Source: CAD feature listing. Evaluate the final solid. Frame: model axes, mm. Face numbers are marked on the shaded views. A direction names the side the tool comes from. Coordinates: 2 decimals unless noted, no trailing zeros. Loops run counter-clockwise (first coordinate to the right, second up) from the corner with the lowest first, then second, coordinate; pieces in that order, holes last. Notation, with made-up numbers: (-24.75, 68) - (-20.75, 68) arc R21 ccw to (-20.75, 105) - close; hole circle Ø2 at (85.5, 78). An arc over 180 degrees is marked (long way). Use one line per item in the form item = value. Start each with the question number.
from build123d import *

# Parameters (mm, degrees)
SKETCH1_R           = 1.5875
SKETCH1_R_2         = 1.1303
BOSS_EXTRUDE1_DEPTH = 7.14375
CUT_EXTRUDE2_DEPTH  = 0.79375


with BuildPart() as part:
    # Sketch1 → Boss-Extrude1 (new body)
    with BuildSketch(Plane.XY):
        Polygon((6.35, 1.5875), (9.525, 1.5875), (9.525, 4.224628752), (9.525, 10.562648806), (7.319307862, 9.683908365), (-11.458663934, 2.097115291), (-11.458663934, -3.175), (9.525, -3.175), (9.525, -1.5875), (6.35, -1.5875), align=None)
        Circle(SKETCH1_R, mode=Mode.SUBTRACT)
        with Locations((-8.918663934, -0.301005903)):
            Circle(SKETCH1_R_2, mode=Mode.SUBTRACT)
        with Locations((6.624646204, 5.978899029)):
            Circle(SKETCH1_R_2, mode=Mode.SUBTRACT)
    extrude(amount=BOSS_EXTRUDE1_DEPTH)

    # Sketch3 → Cut-Extrude2 (cut)
    with BuildSketch(Plane.XY.offset(7.14375)):
        Polygon((-8.345148438, 3.659663992), (-5.450582972, -3.504636938), (9.525, -3.219186714), (9.525, 3.382363055), (6.034120938, 1.971956363), (3.430086515, 8.417167728), align=None)
    extrude(amount=-CUT_EXTRUDE2_DEPTH, mode=Mode.SUBTRACT)


solid = part.part
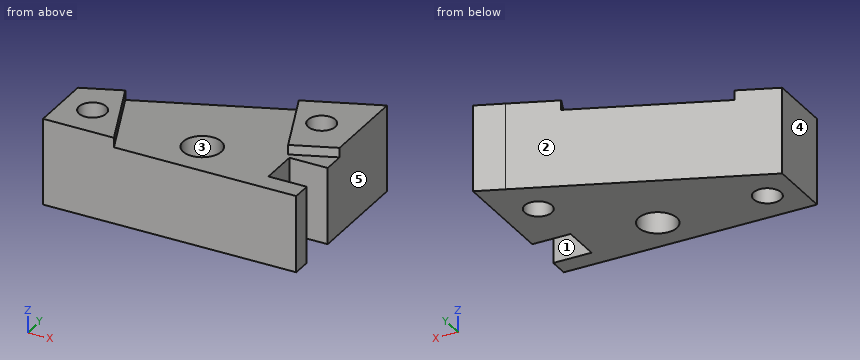
(1) Access query for the marked faces 1 and 2. Directions: +Z, -Z, +X, -X, +Y, -Y. A direction counts if a zero-diameter tool reaches every point of the face in a straight line with its end or side. Return the directions, or none.
(2) Cut plane B-B, the plane y = 0.25. Output: boundary loops of the cut face in (x, z).
(3) Mould query, pull axis X, two halves, no side actions, for the marked faces 3, 4 and 5. Classes: +X half, -X half, draft (parallel to the pull), parting line (faces both ways), or undercut.
(4) Cut plane A-A, the plane z = 6.75. Output: boundary loops of the cut face in (x, y) (3 decimals).
(5) Cut plane D-D, the plane z = 2.25. State how many separate pieces and enclosed holes the cut face has, plus the area to 3 significant figures.
(6) Contact query for flat-ended pins moving along their axis: pin 1 (5.5 mm diameter, centred on x = 4.5, y = 4.5, fed in from +Z); pin 2 (3 mm diameter, centred on x = 2, z = 3, fed in from +Y); pin 3 (1 mm diameter, centred on x = 7.5, z = 4.5, fed in from +Y); pin 4 (2.5 mm diameter, centred on y = 0, z = 3, fed in from +X). Output: stop coordinate, or through.
(7) Material intervals for line 1 (X direction, y = 0, z = 4.25); line 2 (X direction, y = 0.25, z = 1.25); line 3 (Z direction, x = -5.5, y = 0.75), sorted ascending.
Recorded:
q1.face_1 = +Z, -Z, +X
q1.face_2 = +Z, -Z, -X, +Y
q2.outline = (-11.46, 0) - (-9.91, 0) - (-9.91, 7.14) - (-11.46, 7.14) - close; (-7.93, 0) - (-1.57, 0) - (-1.57, 6.35) - (-6.97, 6.35) - (-6.97, 7.14) - (-7.93, 7.14) - close; (1.57, 0) - (6.35, 0) - (6.35, 6.35) - (1.57, 6.35) - close
q3.face_3 = undercut
q3.face_4 = -X half
q3.face_5 = +X half
q4.outline = (-11.459, -3.175) - (-5.584, -3.175) - (-8.239, 3.398) - (-11.459, 2.097) - close; (3.536, 8.155) - (6.034, 1.972) - (9.525, 3.382) - (9.525, 10.563) - (7.319, 9.684) - close; hole circle Ø2.261 at (-8.919, -0.301); hole circle Ø2.261 at (6.625, 5.979)
q5.separate_pieces = 1
q5.enclosed_holes = 3
q5.area = 174 mm²
q6.pin_1 = 7.14
q6.pin_2 = 8.14
q6.pin_3 = 9.96
q6.pin_4 = 6.35
q7.line_1 = -11.46 to -10.01, -7.83 to -1.59, 1.59 to 6.35
q7.line_2 = -11.46 to -9.91, -7.93 to -1.57, 1.57 to 6.35
q7.line_3 = 0 to 6.35
